Source: CAD feature listing. Evaluate the final solid. Frame: model axes, mm. A direction names the side the tool comes from. Coordinates: 2 decimals unless noted, no trailing zeros. Order: outer loops, then holes, each group sorted by start corner. A loop starts at its lowest first (then second) coordinate and runs counter-clockwise, first axis right, second up. Notation, with made-up numbers: (80, 53) - (105, 53) arc R24 cw to (105, 89) - close; hole circle Ø1 at (32.5, -8). An arc over 180 degrees is marked (long way). One line per question, with ' | ' between items.
from build123d import *
from build123d.topology import SkipClean

# Parameters (mm, degrees)
EXTRUDE_1_DEPTH           = 2
FILLET_1_R                = 5
SKETCH_2_R                = 1.65
EXTRUDE_2_DEPTH           = 2
SKETCH_2_2_R              = 1.65
CUT_EXTRUDE_1_DEPTH       = 2
EXTRUDE_3_DEPTH           = 8
REVOLVE_4_ANGLE           = 180
CUT_EXTRUDE_3_DEPTH       = 8
CUT_EXTRUDE_3_DEPTH_BACK  = 50.836922569
CUT_EXTRUDE_4_DEPTH       = 47.549848859
CUT_EXTRUDE_4_DEPTH_BACK  = 47.549848859
EXTRUDE_4_DEPTH           = 8
CUT_EXTRUDE_15_DEPTH      = 2
CUT_EXTRUDE_15_DEPTH_BACK = 51.804237139
SKETCH_16_R               = 8.1
CUT_EXTRUDE_16_DEPTH      = 56.283591172
SKETCH_18_R               = 2.5
CUT_EXTRUDE_17_DEPTH      = 49.721344888
SKETCH_19_R               = 1.65
EXTRUDE_5_DEPTH           = 8
CUT_EXTRUDE_18_DEPTH      = 8


with BuildPart() as part:
    # Sketch 1 → Extrude 1 (new body)
    with BuildSketch(Plane.XY):
        with BuildLine():
            Line((-23.5, 0), (-26.5, 0))
            Line((-26.5, 0), (-26.5, -27.25))
            Line((-26.5, -27.25), (26.5, -27.25))
            Line((26.5, -27.25), (26.5, 0))
            Line((26.5, 0), (23.5, 0))
            ThreePointArc((23.5, 0), (0, -23.5), (-23.5, 0))
        make_face()
    extrude(amount=EXTRUDE_1_DEPTH)

    # Fillet 1
    fillet_1_edges = [part.edges().sort_by_distance(p)[0] for p in [
        (26.5, -27.25, 1),
        (-26.5, -27.25, 1),
    ]]
    fillet(fillet_1_edges, radius=FILLET_1_R)

    # Sketch 2 → Extrude 2 (add)
    with BuildSketch(Plane.XY.offset(2)):
        with Locations((-21.5, -22.25)):
            Circle(SKETCH_2_R)
        with Locations((21.5, -22.25)):
            Circle(SKETCH_2_R)
        Polygon((33.218421053, 0), (26.5, -17.25), (26.5, 0), align=None)
        Polygon((-26.5, -17.25), (-33.218421053, 0), (-26.5, 0), align=None)
    extrude(amount=-EXTRUDE_2_DEPTH)

    # Sketch 2_2 → Cut-Extrude 1 (cut)
    with BuildSketch(Plane.XY.offset(2)):
        with Locations((-21.5, -22.25)):
            Circle(SKETCH_2_2_R)
        with Locations((21.5, -22.25)):
            Circle(SKETCH_2_2_R)
    extrude(amount=-CUT_EXTRUDE_1_DEPTH, mode=Mode.SUBTRACT)

    # Sketch 5 → Extrude 3 (add)
    with BuildSketch(Plane.XY.offset(2)):
        with BuildLine():
            Line((23.5, 0), (32.54831672, 0))
            ThreePointArc((32.54831672, 0), (0, -27.25), (-32.54831672, 0))
            Line((-32.54831672, 0), (-23.5, 0))
            ThreePointArc((-23.5, 0), (0, -23.5), (23.5, 0))
        make_face()
    extrude(amount=EXTRUDE_3_DEPTH)

    # Sketch 8 → Revolve 4 (revolve)
    with BuildSketch(Plane(origin=(0, 0, 0), x_dir=(1, 0, 0), z_dir=(0, 1, 0))):
        with BuildLine():
            add(Edge.make_bspline(
                [(32.54831672, -10), (32.54831672, -19.011252641), (1.892491424, -26.996963713), (0, -27.912632857)],
                knots=[0, 0, 0, 0, 0.940683104, 0.940683104, 0.940683104, 0.940683104], degree=3))
            Line((32.54831672, -10), (23.5, -10))
            ThreePointArc((23.5, -10), (13.428049002, -19.533396273), (0, -23))
            Line((0, -23), (0, -27.912632857))
        make_face()
    revolve(axis=Axis((0, 0, 28), (0, 0, -1)), revolution_arc=REVOLVE_4_ANGLE)

    # Sketch 11 → Cut-Extrude 3 (cut, two sides: drawn at the far end of the back side and taken through both)
    with BuildSketch(Plane(origin=(0, 0, 10), x_dir=(-1, 0, 0), z_dir=(0, 0, -1)).offset(-CUT_EXTRUDE_3_DEPTH_BACK)):
        with BuildLine():
            Line((-30.809155169, -6.185952945), (-32.495321725, -1.856606381))
            ThreePointArc((-32.495321725, -1.856606381), (0, -32.54831672), (32.495321725, -1.856606381))
            Line((32.495321725, -1.856606381), (30.809155169, -6.185952945))
            ThreePointArc((30.809155169, -6.185952945), (0, -27.25), (-30.809155169, -6.185952945))
        make_face()
    extrude(amount=CUT_EXTRUDE_3_DEPTH + CUT_EXTRUDE_3_DEPTH_BACK, mode=Mode.SUBTRACT)

    # Sketch 11_3 → Cut-Extrude 4 (cut, two sides: drawn at the far end of the back side and taken through both)
    with BuildSketch(Plane(origin=(0, 0, 10), x_dir=(-1, 0, 0), z_dir=(0, 0, -1)).offset(-CUT_EXTRUDE_4_DEPTH_BACK)):
        with BuildLine():
            Line((-32.54831672, 0), (-33.218421053, 0))
            Line((-33.218421053, 0), (-32.495321725, -1.856606381))
            ThreePointArc((-32.495321725, -1.856606381), (-32.535065274, -0.928681286), (-32.54831672, 0))
        make_face()
        with BuildLine():
            ThreePointArc((32.54831672, 0), (32.535065274, -0.928681286), (32.495321725, -1.856606381))
            Line((32.495321725, -1.856606381), (33.218421053, 0))
            Line((33.218421053, 0), (32.54831672, 0))
        make_face()
        with BuildLine():
            Line((30.809155169, -6.185952945), (32.495321725, -1.856606381))
            ThreePointArc((32.495321725, -1.856606381), (32.535065274, -0.928681286), (32.54831672, 0))
            ThreePointArc((32.54831672, 0), (31.829370312, -3.13532686), (30.809155169, -6.185952945))
        make_face()
        with BuildLine():
            ThreePointArc((-32.54831672, 0), (-32.535065274, -0.928681286), (-32.495321725, -1.856606381))
            Line((-32.495321725, -1.856606381), (-30.809155169, -6.185952945))
            ThreePointArc((-30.809155169, -6.185952945), (-31.829370312, -3.13532686), (-32.54831672, 0))
        make_face()
    extrude(amount=CUT_EXTRUDE_4_DEPTH + CUT_EXTRUDE_4_DEPTH_BACK, mode=Mode.SUBTRACT)

    # Sketch 13 → Extrude 4 (add)
    with BuildSketch(Plane(origin=(0, 0, 0), x_dir=(1, 0, 0), z_dir=(0, 1, 0))):
        with BuildLine():
            Line((-23.5, 0), (-32.54831672, 0))
            Line((-32.54831672, 0), (-32.54831672, -10))
            add(Edge.make_bspline(
                [(-32.54831672, -10), (-32.54831672, -19.011252636), (-1.892491463, -26.996963703), (-4e-09, -27.912632855)],
                knots=[0, 0, 0, 0, 0.940683104, 0.940683104, 0.940683104, 0.940683104], degree=3))
            add(Edge.make_bspline(
                [(-4e-09, -27.912632855), (1.892491463, -26.996963703), (32.54831672, -19.011252636), (32.54831672, -10)],
                knots=[0, 0, 0, 0, 0.940683104, 0.940683104, 0.940683104, 0.940683104], degree=3))
            Line((32.54831672, -10), (32.54831672, 0))
            Line((32.54831672, 0), (23.5, 0))
            Line((23.5, 0), (23.5, -10))
            ThreePointArc((23.5, -10), (0, -23), (-23.5, -10))
            Line((-23.5, -10), (-23.5, 0))
        make_face()
    extrude(amount=EXTRUDE_4_DEPTH)

    # Sketch 16 → Cut-Extrude 15 (cut, two sides: drawn at the far end of the back side and taken through both)
    with BuildSketch(Plane(origin=(0, 0, 27.912632848), x_dir=(-1, 0, 0), z_dir=(0, 0, -1)).offset(-CUT_EXTRUDE_15_DEPTH_BACK)):
        Circle(SKETCH_16_R)
    extrude(amount=CUT_EXTRUDE_15_DEPTH + CUT_EXTRUDE_15_DEPTH_BACK, mode=Mode.SUBTRACT)

    # Sketch 17 → Cut-Extrude 16 (cut, through all)
    with BuildSketch(Plane(origin=(0, 8, 0), x_dir=(1, 0, 0), z_dir=(0, 1, 0))):
        with BuildLine():
            Line((-6.136694484, -25.912632848), (-1.268857754, -25.912632848))
            Line((-1.268857754, -25.912632848), (-1.268857754, -27.464886901))
            add(Edge.make_bspline(
                [(-1.268857754, -27.464886901), (-2.37160723, -27.10853767), (-4.077764087, -26.58262095), (-6.136694484, -25.912632848)],
                knots=[0.699251463, 0.699251463, 0.699251463, 0.699251463, 0.851241237, 0.851241237, 0.851241237, 0.851241237], degree=3))
        make_face()
        with BuildLine():
            Line((1.268857754, -27.464886901), (1.268857754, -25.912632848))
            Line((1.268857754, -25.912632848), (6.136694484, -25.912632848))
            add(Edge.make_bspline(
                [(6.136694484, -25.912632848), (4.077764087, -26.58262095), (2.37160723, -27.10853767), (1.268857754, -27.464886901)],
                knots=[0.089441867, 0.089441867, 0.089441867, 0.089441867, 0.241431641, 0.241431641, 0.241431641, 0.241431641], degree=3))
        make_face()
    extrude(amount=-CUT_EXTRUDE_16_DEPTH, mode=Mode.SUBTRACT)

    # Sketch 18 → Cut-Extrude 17 (cut, through all)
    with BuildSketch(Plane.XY.offset(2)):
        with Locations((-21.5, -22.25)):
            Circle(SKETCH_18_R)
        with Locations((21.5, -22.25)):
            Circle(SKETCH_18_R)
    extrude(amount=CUT_EXTRUDE_17_DEPTH, mode=Mode.SUBTRACT)

    # Sketch 19 → Extrude 5 (add)
    with SkipClean():  # the faces are left unmerged after this step: merging them gives an invalid solid
        with BuildSketch(Plane(origin=(0, 0, 0), x_dir=(-1, 0, 0), z_dir=(0, 0, -1))):
            with BuildLine():
                Line((26.5, -17.25), (30.809155169, -6.185952945))
                ThreePointArc((30.809155169, -6.185952945), (31.829370312, -3.13532686), (32.54831672, 0))
                Line((32.54831672, 0), (32.54831672, 8))
                Line((32.54831672, 8), (23.5, 8))
                Line((23.5, 8), (23.5, 0))
                ThreePointArc((23.5, 0), (0, -23.5), (-23.5, 0))
                Line((-23.5, 0), (-23.5, 8))
                Line((-23.5, 8), (-32.54831672, 8))
                Line((-32.54831672, 8), (-32.54831672, 0))
                ThreePointArc((-32.54831672, 0), (-31.829370312, -3.13532686), (-30.809155169, -6.185952945))
                Line((-30.809155169, -6.185952945), (-26.5, -17.25))
                Line((-26.5, -17.25), (-26.5, -22.25))
                ThreePointArc((-26.5, -22.25), (-25.035533906, -25.785533906), (-21.5, -27.25))
                Line((-21.5, -27.25), (21.5, -27.25))
                ThreePointArc((21.5, -27.25), (25.035533906, -25.785533906), (26.5, -22.25))
                Line((26.5, -22.25), (26.5, -17.25))
            make_face()
            with Locations(Location((21.5, -22.25, 0), (0, 0, 180))):
                Circle(SKETCH_19_R, mode=Mode.SUBTRACT)
            with Locations(Location((-21.5, -22.25, 0), (0, 0, 180))):
                Circle(SKETCH_19_R, mode=Mode.SUBTRACT)
        extrude(amount=EXTRUDE_5_DEPTH)

    # Sketch 20 → Cut-Extrude 18 (cut)
    with SkipClean():  # the faces are left unmerged after this step: merging them gives an invalid solid
        with BuildSketch(Plane.XY.offset(2)):
            with BuildLine():
                ThreePointArc((19.32782273, -21.012403172), (10.154707599, -25.651983205), (0, -27.25))
                Line((0, -27.25), (21.5, -27.25))
                ThreePointArc((21.5, -27.25), (25.035533906, -25.785533906), (26.5, -22.25))
                Line((26.5, -22.25), (26.5, -17.25))
                Line((26.5, -17.25), (30.809155169, -6.185952945))
                ThreePointArc((30.809155169, -6.185952945), (26.725252476, -13.653221694), (20.870444361, -19.830566244))
                ThreePointArc((20.870444361, -19.830566244), (19.979601548, -20.265462637), (19.32782273, -21.012403172))
            make_face()
            with BuildLine():
                Line((-21.5, -27.25), (0, -27.25))
                ThreePointArc((0, -27.25), (-10.154707599, -25.651983205), (-19.32782273, -21.012403172))
                ThreePointArc((-19.32782273, -21.012403172), (-19.979601548, -20.265462637), (-20.870444361, -19.830566244))
                ThreePointArc((-20.870444361, -19.830566244), (-26.725252476, -13.653221694), (-30.809155169, -6.185952945))
                Line((-30.809155169, -6.185952945), (-26.5, -17.25))
                Line((-26.5, -17.25), (-26.5, -22.25))
                ThreePointArc((-26.5, -22.25), (-25.035533906, -25.785533906), (-21.5, -27.25))
            make_face()
        extrude(amount=-CUT_EXTRUDE_18_DEPTH, mode=Mode.SUBTRACT)


solid = part.part
(1) Set-up query: faces 1 (the cylindrical face through (-0.517, -23.494, 1.126)), 2 (the flat face through (20, -24, -6)), 3 (the flat face through (-20, -24, -6)), 4 (the flat face through (-26.5, -20, -7)). Return all of +Z, -Z, +X, -X, +Y, -Y with unobstructed straight access to the full face (end or side cutting, diameter ignored); none if empty.
Taken from the geometry:
face 1: -Z, +Y | face 2: +Z, +X, -Y | face 3: +Z, -X, -Y | face 4: +Z, -Z, -X, -Y
(2) Material intervals for L1, parallel to Z at x = -24.5, y = -19; L2, parallel to Y at x = 21.5, z = -6.6; L3, parallel to X at y = -19.5, z = 7.5, sorted ascending. Write a range as from..to.
Taken from the geometry:
L1: z = -8..-6 | L2: y = -27.25..-23.9, -20.6..-9.49 | L3: x = -21.27..-13.11, 13.11..21.27
(3) Cut plane A-A (z = -2). Return the cut outline in (x, y), and give its area (3 significant figures).
Taken from the geometry:
outline: (-32.55, 0) arc R33.06 ccw to (-20.87, -19.83) arc R2.5 cw to (-19.33, -21.01) arc R33.06 ccw to (19.33, -21.01) arc R2.5 cw to (20.87, -19.83) arc R33.06 ccw to (32.55, 0) - (32.55, 8) - (23.5, 8) - (23.5, 0) arc R23.5 cw to (-23.5, 0) - (-23.5, 8) - (-32.55, 8) - close | area: 611 mm²
(4) Pin query (flat end, axial travel): P1, Ø10, axis at x = 24.5, z = 14, coming from the -Y side; P2, Ø17, axis at x = 8.5, y = -18.5, coming from the +Z side; P3, Ø17, axis at x = -17.5, y = -20, coming from the +Z side. Return the tip coordinate at first contact, or that it passes through.
Taken from the geometry:
P1: stops at y = -20.75 | P2: stops at z = 23.96 | P3: stops at z = 21.54
(5) Pull-direction query (X, two-part tool) for faces 5 (the flat face through (0, -27.25, -7)), 6 (the cylindrical face through (25.07, -25.75, -6.99)), 7 (the cylindrical face through (-22.716, -23.365, -6.986)); classes: pulls with the +X half, pulls with the -X half, needs draft (parallel to the pull), parting line crosses it, or undercut.
Taken from the geometry:
face 5: needs draft | face 6: pulls with the +X half | face 7: undercut
